Read the model definition and answer for the solid it produces. Units are mm, in the model's axes. A direction names the side the tool comes from. Coordinates: 2 decimals unless noted, no trailing zeros. Write each loop counter-clockwise with the first axis right and the second up, starting at its lowest first coordinate (ties: lowest second). Pieces come first, ordered by that corner, then holes. Notation, with made-up numbers: (-17, 21.5) -> (3, 21.5) arc R16 cw to (3, 45.5) -> close; hole circle Ø9 at (18.25, 49). An arc over 180 degrees is marked (long way). Answer in a Markdown table with one row per item. Add a question column.
Item 1: Section A-A on y = 2.75 is taken. Write down the section's boundary in (x, z), then the cut area to 3 significant figures.
Item 2: Section B-B on y = -1.25 is taken. Write down the section's boundary in (x, z).
Item 3: Given pin 1 Ø1 at (y, z) = (5, -2.5) entering from -X; pin 2 Ø4 at (y, z) = (14.5, -3) entering from +X; pin 3 Ø1.5 at (x, y) = (-3, 16.5) entering from +Z, each flat-ended and moving along its own axis, determine where each tip first touches the part or whether it passes through.
Item 4: Straight lines are drawn through the part: line 1 (Y direction, x = -3, z = 1.75); line 2 (Z direction, x = 0, y = 17.75); line 3 (Z direction, x = 1, y = -4). For each, find the intervals that lie inside material, in ascending order. Write a range as from..to.
Item 5: For a pull along Z with two mould halves and no side action, classify faces 4 (the face through (2.285, -2.255, -3.584)), 5 (the face through (0, 20, 0)), 6 (the face through (-1.724, -3.542, 1.014)) as +Z half, -Z half, draft (parallel to the pull), parting line (faces both ways), or undercut.
Item 6: Which of the six approach directions +Z, -Z, +X, -X, +Y, -Y give full straight-line access (tool end or side, diameter ignored) to faces 1 (the face through (-0.54, 10.07, 2.44)), 2 (the face through (1.74, -3.54, 0.99)), 3 (the face through (2, -5, 2))?
Solid Edge part; units mm, degrees
sketch "Sketch1" plane through (0, 0, 0) normal (0, 0, 1) x (1, 0, 0)
  line L0 (2.5, 0) -> (2.5, 20)
  line L1 (0, 20) -> (2.5, 20)
  line L2 (0, 0) -> (0, 20)
  line L3 (0, 0) -> (0, -5)
  line L4 (0, -5) -> (4.25, -5)
  line L5 (4.25, -5) -> (4.25, 0)
  line L6 (4.25, 0) -> (2.5, 0)
revolve "RevolvedProtrusion1" add sketch "Sketch1" angle 360 about axis through (0, 0, 0) along (0, 1, 0)
sketch "Sketch2" plane through (0, 0, 0) normal (1, 0, 0) x (0, 1, 0)
  line L0 (-5, 2.7915) -> (-2.5, 2.7915)
  line L1 (-0.8883, 0) -> (-2.5, 2.7915)
  line L2 (-5, 0) -> (-0.8883, 0)
  line L3 (-5, 0) -> (-5, 2.7915)
revolve "RevolvedCutout1" cut sketch "Sketch2" angle 360 about axis through (0, -4.5, 0) along (0, 1, 0)
sketch "Sketch3" plane through (0, -5, 0) normal (0, -1, 0) x (0, 0, 1)
  circle A0 centre (0, 0) radius 2.7915
  line L0 (-2, -1.1547) -> (0, -2.3094)
  line L1 (0, -2.3094) -> (2, -1.1547)
  line L2 (2, -1.1547) -> (2, 1.1547)
  line L3 (2, 1.1547) -> (0, 2.3094)
  line L4 (0, 2.3094) -> (-2, 1.1547)
  line L5 (-2, 1.1547) -> (-2, -1.1547)
extrude "Protrusion1" add sketch "Sketch3" against normal up to next
sketch "Sketch4" plane through (0, 0, 0) normal (0, 0, 1) x (1, 0, 0)
  line L0 (-2.3094, -5) -> (0, -5)
  line L1 (0, -5) -> (0, -4.3812)
  line L2 (0, -4.3812) -> (-2.3094, -5)
revolve "RevolvedCutout2" cut sketch "Sketch4" angle 360 about axis through (0, -4.5, 0) along (0, 1, 0)
fillet "Round1" radius 0.2 1 edges at (0, 0, -2.5)
fillet "Round2" radius 0.425 1 edges at (0, -5, -4.25)
chamfer "倒斜角_2" distance 0.3333 angle 45 1 edges at (0, 20, -2.5)
cosmetic_thread "螺纹_3" thread depth 16
Results below:
| question | item | result |
|---|---|---|
| 1 | outline | circle Ø5 at (0, 0) |
| 1 | area | 19.6 mm2 |
| 2 | outline | circle Ø8.5 at (0, 0); hole circle Ø1.25 at (0, 0) |
| 3 | pin 1 | stops at x = -1.5 |
| 3 | pin 2 | stops at x = 2.29 |
| 3 | pin 3 | stops at z = 1.09 |
| 4 | line 1 | y = -5..0 |
| 4 | line 2 | z = -2.5..2.5 |
| 4 | line 3 | z = -4.13..-2, 2..4.13 |
| 5 | face 4 | parting line |
| 5 | face 5 | draft |
| 5 | face 6 | undercut |
| 6 | face 1 | +Y |
| 6 | face 2 | -Y |
| 6 | face 3 | +Z, -Z, +X, -X, -Y |
